Build history of the part. All positions in model axes, mm. Face numbers are marked on the shaded views. A direction names the side the tool comes from. Round coordinates to 2 decimals unless told otherwise and drop trailing zeros. Write each loop counter-clockwise with the first axis right and the second up, starting at its lowest first coordinate (ties: lowest second). Pieces come first, ordered by that corner, then holes.
from build123d import *

# Parameters (mm, degrees)
SKETCH1_R           = 7.5
SKETCH1_R_2         = 4
BOSS_EXTRUDE1_DEPTH = 8
BOSS_EXTRUDE2_START = 1
SKETCH2_R           = 7.5
BOSS_EXTRUDE2_DEPTH = 1
BOSS_EXTRUDE3_DEPTH = 7
BOSS_EXTRUDE4_START = 17.5
SKETCH4_R           = 7.5
BOSS_EXTRUDE4_DEPTH = 17.5
BOSS_EXTRUDE5_START = 2
SKETCH5_R           = 7.5
SKETCH5_R_2         = 2.5
BOSS_EXTRUDE5_DEPTH = 2
SKETCH6_W           = 7
SKETCH6_H           = 1
CUT_EXTRUDE1_DEPTH  = 19.5
FILLET1_R           = 0.2
SKETCH7_W           = 10
SKETCH7_H           = 1
CUT_EXTRUDE2_DEPTH  = 8


with BuildPart() as part:
    # Sketch1 → Boss-Extrude1 (new body)
    with BuildSketch(Plane(origin=(0, 0, 0), x_dir=(0, 0, -1), z_dir=(1, 0, 0))):
        Circle(SKETCH1_R)
        Circle(SKETCH1_R_2, mode=Mode.SUBTRACT)
    extrude(amount=BOSS_EXTRUDE1_DEPTH)

    # Sketch2 → Boss-Extrude2 (add)
    with BuildSketch(Plane.ZY.offset(BOSS_EXTRUDE2_START)):
        Circle(SKETCH2_R)
    extrude(amount=-BOSS_EXTRUDE2_DEPTH)

    # Sketch3 → Boss-Extrude3 (add)
    with BuildSketch(Plane(origin=(0, 0, 0), x_dir=(0, 0, -1), z_dir=(1, 0, 0))):
        with BuildLine():
            Line((-3.771236166, 1.333333333), (3.771236166, 1.333333333))
            ThreePointArc((3.771236166, 1.333333333), (0, 4), (-3.771236166, 1.333333333))
        make_face()
    extrude(amount=BOSS_EXTRUDE3_DEPTH)

    # Sketch4 → Boss-Extrude4 (add)
    with BuildSketch(Plane.ZY.offset(1).offset(BOSS_EXTRUDE4_START)):
        Circle(SKETCH4_R)
        with BuildLine():
            ThreePointArc((1.5, -2), (0, 2.5), (-1.5, -2))
            Line((-1.5, -2), (1.5, -2))
        make_face(mode=Mode.SUBTRACT)
    extrude(amount=-BOSS_EXTRUDE4_DEPTH)

    # Sketch5 → Boss-Extrude5 (add)
    with BuildSketch(Plane.ZY.offset(18.5).offset(BOSS_EXTRUDE5_START)):
        Circle(SKETCH5_R)
        with Locations(Location((0, 0, 0), (0, 0, 233.130102354))):
            Circle(SKETCH5_R_2, mode=Mode.SUBTRACT)
    extrude(amount=-BOSS_EXTRUDE5_DEPTH)

    # Sketch6 → Cut-Extrude1 (cut)
    with BuildSketch(Plane.ZY.offset(20.5)):
        Rectangle(SKETCH6_W, SKETCH6_H)
    extrude(amount=-CUT_EXTRUDE1_DEPTH, mode=Mode.SUBTRACT)

    # Fillet1
    fillet1_edges = [part.edges().sort_by_distance(p)[0] for p in [
        (-9.75, 0.5, -2.449489743),
        (-9.75, 0.5, 2.449489743),
        (-9.75, -0.5, 2.449489743),
        (-9.75, -0.5, -2.449489743),
        (-10.75, 0.5, 3.5),
        (-10.75, -0.5, 3.5),
        (-10.75, -0.5, -3.5),
        (-10.75, 0.5, -3.5),
    ]]
    fillet(fillet1_edges, radius=FILLET1_R)

    # Sketch7 → Cut-Extrude2 (cut)
    with BuildSketch(Plane(origin=(8, 0, 0), x_dir=(0, 0, -1), z_dir=(1, 0, 0))):
        Rectangle(SKETCH7_W, SKETCH7_H)
    extrude(amount=-CUT_EXTRUDE2_DEPTH, mode=Mode.SUBTRACT)


solid = part.part
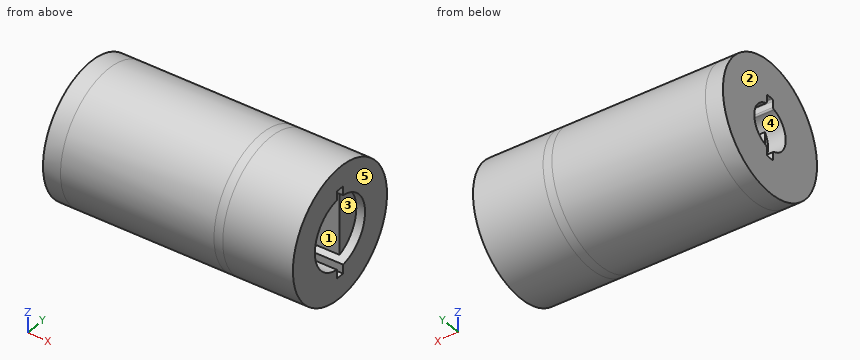
1) Slice it at C-C (y = 0). Write the cut outline in (x, z), plus the area to 3 significant figures.
Results:
outline: (-20.5, -7.5) - (8, -7.5) - (8, -5) - (0, -5) - (0, 5) - (8, 5) - (8, 7.5) - (-20.5, 7.5) - (-20.5, 3.5) - (-1, 3.5) - (-1, -3.5) - (-20.5, -3.5) - close
area: 211 mm2
2) Slice it at D-D (z = 6). Write the cut outline in (x, y).
Results:
outline: (-20.5, -4.5) - (8, -4.5) - (8, 4.5) - (-20.5, 4.5) - close
3) Pin check, flat tips, straight feed: pin 1 Ø0.9 at (y, z) = (1, 0) entering from +X; pin 2 Ø0.8 at (x, z) = (-12.5, -3) entering from +Y; pin 3 Ø1 at (x, z) = (-1, 1.5) entering from -Y. Stop position of each tip, or through.
Results:
pin 1: stops at x = 7
pin 2: stops at y = 7.03
pin 3: stops at y = -7.43
4) Which spindle directions (+Z, -Z, +X, -X, +Y, -Y) get a long thin tool onto all of the face, cutting with end or side? Do the marked faces 3, 4 and 5. Say none if no direction does.
Results:
face 3: +X
face 4: -X
face 5: +Z, -Z, +X, +Y, -Y
5) Wall check: L1, parallel to Y at x = -3.25, z = 0; L2, parallel to X at y = -0.75, z = -2.25; L3, parallel to X at y = 1.75, z = -2.75. Give the ranges that are in metal, low to high.
Results:
L1: y = -7.5 to -2, 2.5 to 7.5
L2: x = -1 to 0
L3: x = -20.5 to 7
6) Slice it at A-A (x = -9). Write the cut outline in (y, z).
Results:
outline: circle Ø15 at (0, 0); hole (-2, -1.5) arc R2.5 ccw to (-0.65, -2.41) arc R0.2 cw to (-0.5, -2.61) - (-0.5, -3.3) arc R0.2 ccw to (-0.3, -3.5) - (0.3, -3.5) arc R0.2 ccw to (0.5, -3.3) - (0.5, -2.61) arc R0.2 cw to (0.65, -2.41) arc R2.5 ccw to (0.65, 2.41) arc R0.2 cw to (0.5, 2.61) - (0.5, 3.3) arc R0.2 ccw to (0.3, 3.5) - (-0.3, 3.5) arc R0.2 ccw to (-0.5, 3.3) - (-0.5, 2.61) arc R0.2 cw to (-0.65, 2.41) arc R2.5 ccw to (-2, 1.5) - close
7) Mould opens along Y. For the marked faces 1 and 2 say: released by +Y, released by -Y, zero draft, split by the parting line, or undercut.
Results:
face 1: undercut
face 2: zero draft
8) Slice it at B-B (z = 0). Write the cut outline in (x, y), plus the area to 3 significant figures.
Results:
outline: (-20.5, -7.5) - (8, -7.5) - (8, -4) - (0, -4) - (0, 1.33) - (7, 1.33) - (7, 4) - (8, 4) - (8, 7.5) - (-20.5, 7.5) - (-20.5, 2.5) - (-1, 2.5) - (-1, -2) - (-18.5, -2) - (-18.5, -2.5) - (-20.5, -2.5) - close
area: 293 mm2
